Build history of the part. All positions in model axes, mm. A direction names the side the tool comes from. Round coordinates to 2 decimals unless told otherwise and drop trailing zeros. Write each loop counter-clockwise with the first axis right and the second up, starting at its lowest first coordinate (ties: lowest second). Pieces come first, ordered by that corner, then holes. Notation, with made-up numbers: (32, 22) -> (49, 22) arc R26 cw to (49, 61) -> close; hole circle Ø4 at (11.25, 52). An arc over 180 degrees is marked (long way). Return JSON: item names as keys, results as strings.
from build123d import *

# Parameters (mm, degrees)
BOSS_EXTRU_1_DEPTH              = 90
CONG_1_R                        = 10
CHANFREIN1_SIZE                 = 5
CONG_2_R                        = 2
ENL_V_MAT_EXTRU_1_DEPTH         = 2
R_P_TITION_LIN_AIRE1_COUNT      = 4
R_P_TITION_LIN_AIRE1_PITCH      = 20.828705533
R_P_TITION_LIN_AIRE1_COUNT_DIR2 = 2
R_P_TITION_LIN_AIRE1_PITCH_DIR2 = 19.691351592


with BuildPart() as part:
    # Esquisse1 → Boss.-Extru.1 (new body)
    with BuildSketch(Plane.XY):
        Polygon((-4.05, 2.83584053), (-4.05, 102.83584053), (4.05, 102.83584053), (4.05, 2.83584053), (36.816081772, 25.778897984), (36.816081772, 45.778897984), (35.216081772, 45.778897984), (35.216081772, 27.1001151), (6.05, 6.677804784), (6.05, 104.83584053), (-6.05, 104.83584053), (-6.05, 4.83584053), (-64.05, 4.83584053), (-64.05, 16.888959942), (-66.05, 16.888959942), (-66.05, 2.83584053), (-6.05, 2.83584053), align=None)
    extrude(amount=BOSS_EXTRU_1_DEPTH)

    # Congé1
    cong_1_edges = [part.edges().sort_by_distance(p)[0] for p in [
        (-66.05, 2.83584053, 45),
        (-64.05, 4.83584053, 45),
        (-6.05, 4.83584053, 45),
        (6.05, 6.677804784, 45),
        (35.216081772, 27.1001151, 45),
    ]]
    fillet(cong_1_edges, radius=CONG_1_R)

    # Chanfrein1
    chanfrein1_edges = [part.edges().sort_by_distance(p)[0] for p in [
        (36.016081772, 45.778897984, 0),
        (36.016081772, 45.778897984, 90),
        (-65.05, 16.888959942, 0),
        (-65.05, 16.888959942, 90),
    ]]
    chamfer(chanfrein1_edges, length=CHANFREIN1_SIZE)

    # Congé2
    cong_2_edges = [part.edges().sort_by_distance(p)[0] for p in [
        (36.816081772, 25.778897984, 45),
        (4.05, 2.83584053, 45),
        (36.016081772, 40.778897984, 90),
        (36.016081772, 40.778897984, 0),
        (36.016081772, 45.778897984, 5),
        (36.016081772, 45.778897984, 85),
        (-64.805502489, 11.888959942, 90),
        (-65.05, 16.888959942, 85),
        (-64.805502489, 11.888959942, 0),
        (-65.05, 16.888959942, 5),
        (6.05, 104.83584053, 45),
        (-6.05, 104.83584053, 45),
        (-4.05, 2.83584053, 45),
    ]]
    fillet(cong_2_edges, radius=CONG_2_R)

    # Esquisse2 → Enlèv. mat.-Extru.1 (cut)
    with BuildSketch(Plane.XZ.offset(-2.83584053)):
        Polygon((-49.883487215, 12.442815588), (-42.812419404, 19.5138834), (-35.741351592, 12.442815588), (-42.812419404, 5.371747776), align=None)
    enl_v_mat_extru_1 = extrude(amount=-ENL_V_MAT_EXTRU_1_DEPTH, mode=Mode.SUBTRACT)

    # Répétition linéaire1: Enl_v. mat.-Extru.1 4 × 2
    with Locations(*[(j * R_P_TITION_LIN_AIRE1_PITCH_DIR2, 0, i * R_P_TITION_LIN_AIRE1_PITCH) for i in range(R_P_TITION_LIN_AIRE1_COUNT) for j in range(R_P_TITION_LIN_AIRE1_COUNT_DIR2) if (i, j) != (0, 0)]):
        add(enl_v_mat_extru_1, mode=Mode.SUBTRACT)


solid = part.part
Q1. Saw through at C-C on z = 15.5. Count the separate pieces of the cut face and the enclosed holes in it, then the cut area to 3 significant figures.
Verdict:
{"separate pieces": "3", "enclosed holes": "0", "area": "741 mm²"}
Q2. Saw through at B-B on y = 72. List the corners of the cut face in (x, z).
Verdict:
{"outline": "(-6.05, 0) -> (-4.05, 0) -> (-4.05, 90) -> (-6.05, 90) -> close; (4.05, 0) -> (6.05, 0) -> (6.05, 90) -> (4.05, 90) -> close"}
Q3. 3-axis set-ups, long thin cutter, end or side, ignore diameter. For faces 1 (the flat face through (-46.397, 3.822, 15.929)), 2 (the cylindrical face through (-61.043, 7.687, 45.63)), 3 (the flat face through (-66.05, 15, 44)), 4 (the flat face through (-4.05, 53, 44)), 5 (the flat face through (-64.89, 14.42, 87.47)): which of +Z, -Z, +X, -X, +Y, -Y reach the whole face in a straight line?
Verdict:
{"face 1": "+Y, -Y", "face 2": "+Z, -Z, +Y", "face 3": "+Z, -Z, -X, +Y, -Y", "face 4": "+Z, -Z, -Y", "face 5": "+Z, -X, +Y"}
Q4. Pin check, flat tips, straight feed: pin 1 Ø2 at (x, z) = (10, 48) entering from -Y; pin 2 Ø3 at (y, z) = (73.5, 78.5) entering from +X; pin 3 Ø0.8 at (x, z) = (36.5, 54.5) entering from +Y. Stop position of each tip, or through.
Verdict:
{"pin 1": "stops at y = 6.3", "pin 2": "stops at x = 6.05", "pin 3": "stops at y = 45.78"}
Q5. Saw through at A-A on y = 38. List the corners of the cut face in (x, z), then the cut area to 3 significant figures.
Verdict:
{"outline": "(-6.05, 0) -> (-4.05, 0) -> (-4.05, 90) -> (-6.05, 90) -> close; (4.05, 0) -> (6.05, 0) -> (6.05, 90) -> (4.05, 90) -> close; (35.22, 0) -> (36.82, 0) -> (36.82, 90) -> (35.22, 90) -> close", "area": "504 mm²"}
Q6. Wall check: L1, parallel to X at y = 35, z = 18; L2, parallel to X at y = 46, z = 48.5. Give the ranges that are in metal, low to high.
Verdict:
{"L1": "x = -6.05 to -4.05, 4.05 to 6.05, 35.22 to 36.82", "L2": "x = -6.05 to -4.05, 4.05 to 6.05"}
Q7. Saw through at D-D on x = -27.5. List the corners of the cut face in (y, z), then the cut area to 3 significant figures.
Verdict:
{"outline": "(2.84, 0) -> (4.84, 0) -> (4.84, 9.75) -> (2.84, 9.75) -> close; (2.84, 15.13) -> (4.84, 15.13) -> (4.84, 30.58) -> (2.84, 30.58) -> close; (2.84, 35.96) -> (4.84, 35.96) -> (4.84, 51.41) -> (2.84, 51.41) -> close; (2.84, 56.79) -> (4.84, 56.79) -> (4.84, 72.24) -> (2.84, 72.24) -> close; (2.84, 77.62) -> (4.84, 77.62) -> (4.84, 90) -> (2.84, 90) -> close", "area": "137 mm²"}
Q8. Two-plate mould, pull along Z, no slides. Class faces 6 (the flat face through (4.2, 42.7, 0)), 7 (the flat face through (-46.3, 3.82, 8.86)), 8 (the flat face through (26.43, 20.95, 44.37)): +Z half, -Z half, draft (parallel to the pull), parting line (faces both ways), or undercut.
Verdict:
{"face 6": "-Z half", "face 7": "undercut", "face 8": "draft"}
